Model file for the job. Use its own axes, mm. Give positions to 0.01 mm unless a question says otherwise; leave off trailing zeros. Write each loop counter-clockwise with the first axis right and the second up, starting at its lowest first coordinate (ties: lowest second). Pieces come first, ordered by that corner, then holes. Notation, with made-up numbers: (80.5, 35.5) - (135.5, 35.5) arc R34 ccw to (135.5, 71.5) - close; hole circle Ø4 at (-39, 13.5). An arc over 180 degrees is marked (long way). Use CSV: the item, a comma, the result in double quotes.
from build123d import *

# Parameters (mm, degrees)
ESBO_O2_R                     = 5
RESSALTO_EXTRUS_O2_DEPTH      = 3.5
CHANFRO1_SIZE                 = 0.5
CHANFRO1_SIZE2                = 4.072173214
RESSALTO_EXTRUS_O3_DEPTH      = 4
RESSALTO_EXTRUS_O3_DEPTH_BACK = 1
ESBO_O3_R                     = 1.5
ESBO_O4_R                     = 1.75
RESSALTO_EXTRUS_O4_DEPTH      = 1
CHANFRO2_SIZE                 = 0.5
CHANFRO2_SIZE2                = 0.714074003
FILETE2_R                     = 1
FILETE3_R                     = 2


with BuildPart() as part:
    # Esboço2 → Ressalto-extrusão2 (new body)
    with BuildSketch(Plane(origin=(0, 0, 0), x_dir=(1, 0, 0), z_dir=(0, 1, 0))):
        with Locations(Location((0, 0, 0), (0, 0, 270))):
            Circle(ESBO_O2_R)
    extrude(amount=RESSALTO_EXTRUS_O2_DEPTH)

    # Chanfro1
    chanfro1_edges = [part.edges().sort_by_distance(p)[0] for p in [
        (0, 3.5, -5),
    ]]
    chanfro1_side = [part.faces().sort_by_distance(p)[0] for p in [
        (0, 1.75, -5),
    ]]
    chamfer(chanfro1_edges, length=CHANFRO1_SIZE, length2=CHANFRO1_SIZE2, reference=chanfro1_side[0])

    # Esboço3 → Ressalto-extrusão3 (add, two sides: drawn at the far end of the back side and taken through both)
    with BuildSketch(Plane(origin=(0, 3.5, 0), x_dir=(1, 0, 0), z_dir=(0, 1, 0)).offset(-RESSALTO_EXTRUS_O3_DEPTH_BACK)):
        with Locations(Location((0, 0, 0), (0, 0, 270))):
            Circle(ESBO_O3_R)
    extrude(amount=RESSALTO_EXTRUS_O3_DEPTH + RESSALTO_EXTRUS_O3_DEPTH_BACK)

    # Esboço4 → Ressalto-extrusão4 (add)
    with BuildSketch(Plane(origin=(0, 7.5, 0), x_dir=(1, 0, 0), z_dir=(0, 1, 0))):
        with Locations(Location((0, 0, 0), (0, 0, 270))):
            Circle(ESBO_O4_R)
    extrude(amount=RESSALTO_EXTRUS_O4_DEPTH)

    # Chanfro2
    chanfro2_edges = [part.edges().sort_by_distance(p)[0] for p in [
        (0, 8.5, -1.75),
    ]]
    chanfro2_side = [part.faces().sort_by_distance(p)[0] for p in [
        (0, 8, -1.75),
    ]]
    chamfer(chanfro2_edges, length=CHANFRO2_SIZE, length2=CHANFRO2_SIZE2, reference=chanfro2_side[0])

    # Filete2
    # the kernel refuses this fillet: 1 mm, written as the material it takes off along each edge
    with BuildSketch(Plane(origin=(0, 8, 0), x_dir=(0, 0, 1), z_dir=(-1, 0, 0))) as filete2_piece_1:
        with BuildLine():
            CenterArc((1.75 - FILETE2_R, -FILETE2_R * 0.520567050552), FILETE2_R, 0, 55)
            Line((1.75 - FILETE2_R * 0.426423563649, FILETE2_R * 0.298584993737), (1.75, 0))
            Line((1.75, 0), (1.75, -FILETE2_R * 0.520567050552))
        make_face()
    revolve(axis=Axis((0, 8, 0), (0, 1, 0)), mode=Mode.SUBTRACT)

    # Filete3
    # the kernel refuses this fillet: 2 mm, written as the material it takes off along each edge
    with BuildSketch(Plane(origin=(0, 8.5, 0), x_dir=(0, 0, 1), z_dir=(-1, 0, 0))) as filete3_piece_1:
        with BuildLine():
            CenterArc((0.448881049, -2), FILETE3_R, 64.065224384, 25.934775616)
            Line((0.448881049, 0), (0.448881049, 0.04))
            Line((0.448881049, 0.04), (1.035925997, 0.04))
            Line((1.035925997, 0.04), (1.058869054, 0.032766082))
            ThreePointArc((1.058869054, 0.032766082), (1.202694274, -0.067941421), (1.341070344, -0.165443306))
            Line((1.341070344, -0.165443306), (1.323576436, -0.201415006))
        make_face()
    revolve(axis=Axis((0, 8.5, 0), (0, 1, 0)), mode=Mode.SUBTRACT)


solid = part.part
(1) Flat gauge pins, fed straight in: P1, Ø2, axis at x = 0.5, y = 4.5, coming from the +Z side; P2, Ø3, axis at x = 0, y = 7.5, coming from the +Z side; P3, Ø4, axis at y = 6.5, z = 2, coming from the -X side. Where does each tip first touch, or does it go through?
Checked values:
P1,"stops at z = 1.5"
P2,"stops at z = 1.75"
P3,"stops at x = -1.73"
(2) Pull direction Y, two halves, no side cores. Call faces 1 (the face through (-4.88, 1.48, -1.08)), 2 (the face through (0.45, 5.44, 1.43)), 3 (the face through (0, 8.5, 0)): released by +Y, released by -Y, zero draft, split by the parting line, or undercut.
Checked values:
face 1,"zero draft"
face 2,"undercut"
face 3,"released by +Y"
(3) Wall check: probe 1 along X at (y, z) = (6, 0); probe 2 along Y at (x, z) = (0.5, 0.75); probe 3 along Y at (x, z) = (2, -3). Give the ranges that are in metal, low to high. Write a range as [from, to].
Checked values:
probe 1,"x = [-1.5, 1.5]"
probe 2,"y = [0, 8.45]"
probe 3,"y = [0, 3.17]"
(4) Saw through at A-A, the plane y = 4. List the corners of the cut face in (x, z), then the cut area to 3 significant figures.
Checked values:
outline,"circle Ø3 at (0, 0)"
area,"7.07 mm^2"
